Model file for the job. Use its own axes, mm. A direction names the side the tool comes from. Coordinates: 2 decimals unless noted, no trailing zeros. Write each loop counter-clockwise with the first axis right and the second up, starting at its lowest first coordinate (ties: lowest second). Pieces come first, ordered by that corner, then holes. Notation, with made-up numbers: (-13.75, 87) - (-0.75, 87) arc R24 cw to (-0.75, 124) - close; hole circle Ø10 at (-25, 75.25). An arc over 180 degrees is marked (long way). Put each result on its own line as item: value. Start each with the question number.
1. Pull direction X, two halves, no side cores. Call faces 6 (the face through (0, 2, 3)), 7 (the face through (-99.06, 3, 6)), 8 (the face through (-95.93, -2.75, -12.4)), 9 (the face through (-8.89, -6.2, -2)): released by +X, released by -X, zero draft, split by the parting line, or undercut.
2. Saw through at A-A, the plane x = -21.5. Write the cut outline in (y, z) (3 decimals), plus the area to 3 significant figures.
3. Drill centre lines: L1, parallel to X at y = -4, z = 7; L2, parallel to X at y = 5.5, z = -9; L3, parallel to X at y = 13.5, z = -5.5. Where is each one in solid material? Low to high. Write a range as from..to.
4. Which spindle directions (+Z, -Z, +X, -X, +Y, -Y) get a long thin tool onto all of the face, cutting with end or side? Do faces 1 (the face through (-50.09, -3.1, 0.69)), 2 (the face through (-100.35, -1.38, -6.2)), 3 (the face through (-6.35, 3, 6)), 4 (the face through (-4.47, -2.75, -12.4)), 5 (the face through (-101.6, -2, 3)). Say none if no direction does.
5. Drop flat-ended pins along their axis: P1, Ø1.5, axis at x = -50.5, z = 5.5, coming from the -Y side; P2, Ø6, axis at x = -71, z = -3.5, coming from the -Y side; P3, Ø1, axis at y = -12, z = -1.5, coming from the +X side. Give the stop position or say it passes through.
```python
from build123d import *

# Parameters (mm, degrees)
SKETCH2_R               = 3.175
CUT_EXTRUDE1_DEPTH      = 1
CUT_EXTRUDE1_DEPTH_BACK = 102.6


with BuildPart() as part:
    # Sketch1 → Revolve1 (revolve)
    with BuildSketch(Plane.XY):
        Polygon((0, 0), (0, 6.35), (-2.54, 6.35), (-2.54, 12.7), (-6.35, 12.7), (-6.35, 6.35), (-8.89, 6.35), (-8.89, 9.525), (-33.67488639, 9.525), (-33.67488639, 6.35), (-36.21488639, 6.35), (-36.21488639, 15.875), (-46.531378447, 15.875), (-46.531378447, 6.35), (-92.71, 6.35), (-92.71, 12.7), (-99.06, 12.7), (-99.06, 6.35), (-101.6, 6.35), (-101.6, 0), align=None)
    revolve(axis=Axis((0, 0, 0), (1, 0, 0)))

    # Sketch2 → Cut-Extrude1 (cut, two sides)
    with BuildSketch(Plane(origin=(0, 0, 0), x_dir=(0, 0, -1), z_dir=(1, 0, 0))) as cut_extrude1_sk:
        Circle(SKETCH2_R)
    extrude(amount=CUT_EXTRUDE1_DEPTH, mode=Mode.SUBTRACT)
    extrude(cut_extrude1_sk.sketch, amount=-CUT_EXTRUDE1_DEPTH_BACK, mode=Mode.SUBTRACT)


solid = part.part
```
Final values:
1. face 6: released by +X
1. face 7: released by -X
1. face 8: zero draft
1. face 9: undercut
2. outline: circle Ø19.05 at (0, 0); hole circle Ø6.35 at (0, 0)
2. area: 253 mm²
3. L1: x = -99.06..-92.71, -46.53..-36.21, -33.67..-8.89, -6.35..-2.54
3. L2: x = -99.06..-92.71, -46.53..-36.21, -6.35..-2.54
3. L3: x = -46.53..-36.21
4. face 1: +X, -X
4. face 2: -X
4. face 3: none
4. face 4: +X
4. face 5: +Z, -Z, -X, +Y, -Y
5. P1: stops at y = -4.21
5. P2: stops at y = -6.33
5. P3: stops at x = -2.54
